Input: part model. Units: mm. Frame: model coordinates. A direction names the side the tool comes from. Give positions to 0.01 mm unless a question says otherwise; leave off trailing zeros. Loops run counter-clockwise (first coordinate to the right, second up) from the corner with the lowest first, then second, coordinate; pieces in that order, holes last. Notation, with made-up numbers: (13, 31) -> (27, 31) arc R38 cw to (27, 70) -> close; hole circle Ø1 at (-20, 30). An arc over 180 degrees is marked (long way). Answer in a Markdown table with one row per item. Add a question column.
```python
from build123d import *

# Parameters (mm, degrees)
SKETCH1_R           = 3
BOSS_EXTRUDE1_DEPTH = 2
BOSS_EXTRUDE2_DEPTH = 6
SKETCH3_W           = 5
SKETCH3_H           = 7
CUT_EXTRUDE1_DEPTH  = 3


with BuildPart() as part:
    # Sketch1 → Boss-Extrude1 (new body)
    with BuildSketch(Plane(origin=(0, 0, 0), x_dir=(1, 0, 0), z_dir=(0, 1, 0))):
        with BuildLine():
            Line((6, 6), (-6, 6))
            ThreePointArc((-6, 6), (-12, 0), (-6, -6))
            Line((-6, -6), (-1.5, -6))
            Line((-1.5, -6), (-1.5, -4))
            Line((-1.5, -4), (6, -4))
            Line((6, -4), (6, 6))
        make_face()
        with Locations((-6, 0)):
            Circle(SKETCH1_R, mode=Mode.SUBTRACT)
    extrude(amount=BOSS_EXTRUDE1_DEPTH)

    # Sketch2 → Boss-Extrude2 (add)
    with BuildSketch(Plane(origin=(6, 0, 0), x_dir=(0, 0, -1), z_dir=(1, 0, 0))):
        with BuildLine():
            Line((4, 2), (4, 4))
            ThreePointArc((4, 4), (1, 7), (-2, 4))
            Line((-2, 4), (-2, 2))
            Line((-2, 2), (-4, 2))
            Line((-4, 2), (-4, 4))
            ThreePointArc((-4, 4), (1, 9), (6, 4))
            Line((6, 4), (6, 2))
            Line((6, 2), (4, 2))
        make_face()
    extrude(amount=-BOSS_EXTRUDE2_DEPTH)

    # Sketch3 → Cut-Extrude1 (cut)
    with BuildSketch(Plane.ZY):
        with Locations((1.5, 5.5)):
            Rectangle(SKETCH3_W, SKETCH3_H)
    extrude(amount=-CUT_EXTRUDE1_DEPTH, mode=Mode.SUBTRACT)


solid = part.part
```
1) Section A-A on z = -0.25. Output: boundary loops of the cut face in (x, y), and give its area (3 significant figures).
2) Reachability of faces 4 (the face through (1, 8, -1)), 5 (the face through (3, 1.5, 4)), 6 (the face through (0, 6, -4)), 7 (the face through (5, 3, 2)) from +Z, -Z, +X, -X, +Y, -Y: full face, straight path, thin tool, end or side. Return the list, or none.
3) Section B-B on y = 1.5. Output: boundary loops of the cut face in (x, z).
4) Pull-direction query (Y, two-part tool) for faces 1 (the face through (3.709, 6.796, -2.088)), 2 (the face through (3.709, 8.735, -2.606)), 3 (the face through (-1.5, 1, 5)); classes: +Y half, -Y half, draft (parallel to the pull), parting line (faces both ways), or undercut.
5) Material intervals for line 1 along X through (y, z) = (1.45, 0); line 2 along Z through (x, y) = (-6, 0.5); line 3 along Y through (x, z) = (-8, 5), sorted ascending.
6) Pin query (flat end, axial travel): pin 1 (0.6 mm diameter, centred on y = 0.5, z = 5, fed in from +X); pin 2 (1 mm diameter, centred on x = 4.5, y = 2.5, fed in from +Z); pin 3 (4 mm diameter, centred on y = 5, z = 1.5, fed in from -X). Return the tip coordinate at first contact, or that it passes through.
7) Section D-D on y = 6.5. Output: boundary loops of the cut face in (x, z).
8) Section C-C on x = -7.75. Output: boundary loops of the cut face in (y, z).
Working result:
| question | item | result |
|---|---|---|
| 1 | outline | (-11.99, 0) -> (-8.99, 0) -> (-8.99, 2) -> (-11.99, 2) -> close; (-3.01, 0) -> (6, 0) -> (6, 2) -> (-3.01, 2) -> close; (3, 6.9) -> (6, 6.9) -> (6, 8.94) -> (3, 8.94) -> close |
| 1 | area | 30.1 mm2 |
| 2 | face 4 | +Z, -X, +Y |
| 2 | face 5 | +Z, +X, +Y, -Y |
| 2 | face 6 | +Z, -Z, -X, +Y |
| 2 | face 7 | +X, -X |
| 3 | outline | (-6, -6) -> (6, -6) -> (6, 4) -> (-1.5, 4) -> (-1.5, 6) -> (-6, 6) arc R6 ccw to start; hole circle Ø6 at (-6, 0) |
| 4 | face 1 | undercut |
| 4 | face 2 | +Y half |
| 4 | face 3 | draft |
| 5 | line 1 | x = -12 to -9, -3 to 6 |
| 5 | line 2 | z = -6 to -3, 3 to 6 |
| 5 | line 3 | y = 0 to 2 |
| 6 | pin 1 | stops at x = -1.5 |
| 6 | pin 2 | stops at z = 4 |
| 6 | pin 3 | stops at x = 3 |
| 7 | outline | (0, -5.33) -> (6, -5.33) -> (6, -2.66) -> (0, -2.66) -> close; (3, 0.66) -> (6, 0.66) -> (6, 3.33) -> (3, 3.33) -> close |
| 8 | outline | (0, -5.74) -> (2, -5.74) -> (2, -2.44) -> (0, -2.44) -> close; (0, 2.44) -> (2, 2.44) -> (2, 5.74) -> (0, 5.74) -> close |
